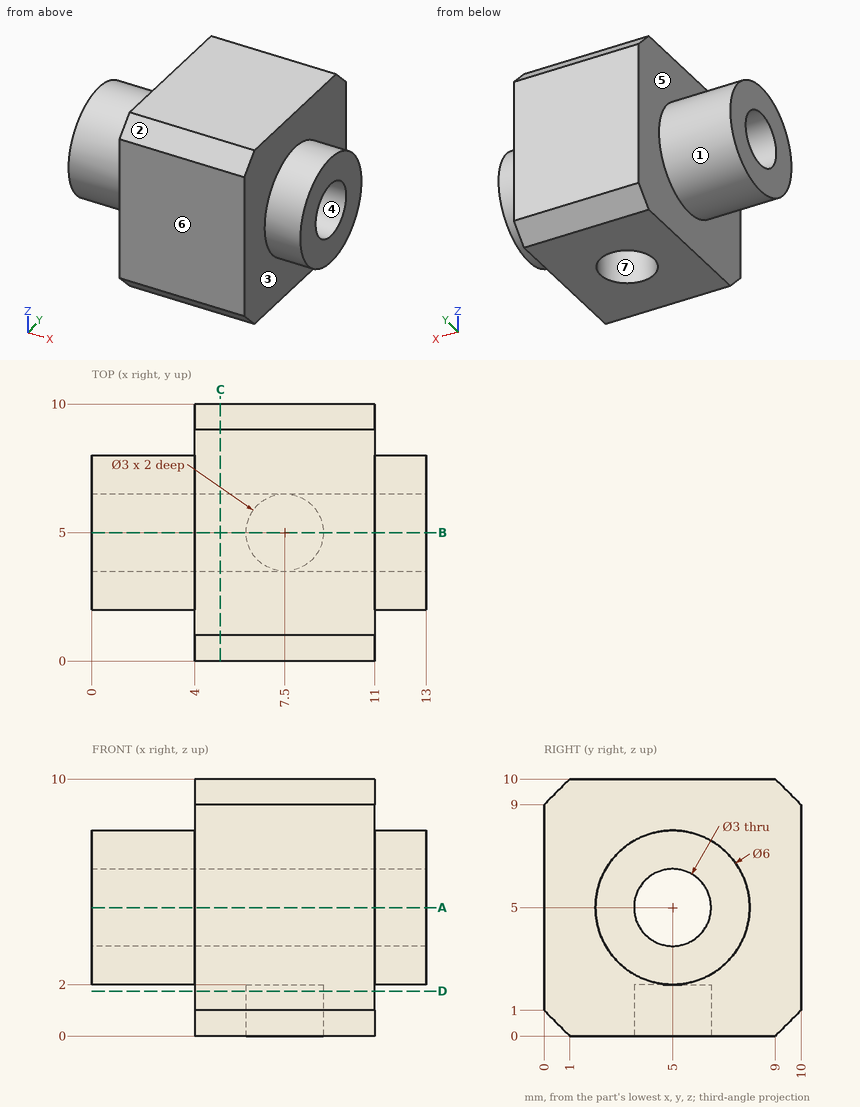
The figure shows three views and two pictorial views of one solid part (mm, origin at its lowest corner). Answer the questions. A direction names the side the tool comes from. Coordinates: 2 decimals unless noted, no trailing zeros. Order: outer loops, then holes, each group sorted by start corner. A loop starts at its lowest first (then second) coordinate and runs counter-clockwise, first axis right, second up.
Q1. A cutting plane is placed at C-C, the plane x = 5. Write down the section's boundary in (y, z).
Q2. For a pull along Y with two mould halves and no side action, classify the marked faces 4, 5, 6 and 7 as pulls with the +Y half, pulls with the -Y half, needs draft (parallel to the pull), parting line crosses it, or undercut.
Q3. Which of the six approach directions +Z, -Z, +X, -X, +Y, -Y give full straight-line access (tool end or side, diameter ignored) to the marked faces 1, 2 and 3?
Q4. Given P1, Ø2.5, axis at y = 5, z = 5, coming from the +X side; P2, Ø2, axis at x = 2.5, y = 2, coming from the +Z side, each flat-ended and moving along its own axis, determine where each tip first touches the part or whether it passes through.
Q5. A cutting plane is placed at B-B, the plane y = 5. Write down the section's boundary in (x, z), and give its area (3 significant figures).
Q6. A cutting plane is placed at D-D, the plane z = 1.75. Write down the section's boundary in (x, y).
Q7. A cutting plane is placed at A-A, the plane z = 5. Write down the section's boundary in (x, y).
Q8. Consider line 1 (Y direction, x = 5.25, z = 5); line 2 (Y direction, x = 1.5, z = 4); line 3 (X direction, y = 9.25, z = 1.75). Determine where each line is inside the solid, lowest interval first.
Answers follow:
1. outline: (0, 1) - (1, 0) - (9, 0) - (10, 1) - (10, 9) - (9, 10) - (1, 10) - (0, 9) - close; hole circle Ø3 at (5, 5)
2. face 4: undercut
2. face 5: needs draft
2. face 6: pulls with the -Y half
2. face 7: undercut
3. face 1: -X
3. face 2: +Z, +X, -X, -Y
3. face 3: +X
4. P1: passes through
4. P2: stops at z = 7.24
5. outline: (0, 2) - (4, 2) - (4, 0) - (6, 0) - (6, 2) - (9, 2) - (9, 0) - (11, 0) - (11, 2) - (13, 2) - (13, 3.5) - (0, 3.5) - close; (0, 6.5) - (13, 6.5) - (13, 8) - (11, 8) - (11, 10) - (4, 10) - (4, 8) - (0, 8) - close
5. area: 61.0 mm2
6. outline: (4, 0) - (11, 0) - (11, 10) - (4, 10) - close; hole circle Ø3 at (7.5, 5)
7. outline: (0, 2) - (4, 2) - (4, 0) - (11, 0) - (11, 2) - (13, 2) - (13, 3.5) - (0, 3.5) - close; (0, 6.5) - (13, 6.5) - (13, 8) - (11, 8) - (11, 10) - (4, 10) - (4, 8) - (0, 8) - close
8. line 1: y = 0 to 3.5, 6.5 to 10
8. line 2: y = 2.17 to 3.88, 6.12 to 7.83
8. line 3: x = 4 to 11
